Source: CAD feature listing. Evaluate the final solid. Frame: model axes, mm. Coordinates: 2 decimals unless noted, no trailing zeros. Order: outer loops, then holes, each group sorted by start corner. A loop starts at its lowest first (then second) coordinate and runs counter-clockwise, first axis right, second up. Notation, with made-up numbers: (21, -37.75) -> (44, -37.75) arc R20 ccw to (44, -27.75) -> close; hole circle Ø7 at (-6, 30). An arc over 180 degrees is marked (long way). Write item = value, one per line. Start each with the question number.
Item 1: Ray query, line 1 along X through (y, z) = (17.5, 0.65); line 2 along X through (y, z) = (18, 2.1). Return the intervals inside material, ascending. Write a range as [from, to].
Item 2: Contact query for flat-ended pins moving along their axis: pin 1 (6 mm diameter, centred on x = -17, y = 13, fed in from -Z); pin 2 (0.8 mm diameter, centred on y = 0, z = 2, fed in from +X); pin 3 (1.4 mm diameter, centred on x = 21, z = 1, fed in from -Y); pin 4 (1.4 mm diameter, centred on x = -22, z = 1.5, fed in from -Y). Output: stop coordinate, or through.
Item 3: Section query B-B (y = 21). Output: boundary loops of the cut face in (x, z), then the cut area to 3 significant figures.
Item 4: Section query A-A (z = 0.6). Output: boundary loops of the cut face in (x, y).
Item 5: Section query D-D (y = -0.5). Output: boundary loops of the cut face in (x, z), then the cut area to 3 significant figures.
Item 6: Section query C-C (x = -17). Output: boundary loops of the cut face in (y, z), then the cut area to 3 significant figures.
```python
from build123d import *

# Parameters (mm, degrees)
CROQUIS1_R              = 25
SALIENTE_EXTRUIR1_DEPTH = 2.8
CROQUIS2_W              = 2.8
CROQUIS2_H              = 18
CORTAR_EXTRUIR1_DEPTH   = 3.8
MATRIZC1_COUNT          = 4


with BuildPart() as part:
    # Croquis1 → Saliente-Extruir1 (new body)
    with BuildSketch(Plane.XY):
        Circle(CROQUIS1_R)
    extrude(amount=SALIENTE_EXTRUIR1_DEPTH)

    # Croquis2 → Cortar-Extruir1 (cut, through all)
    with BuildSketch(Plane.XY):
        with Locations((0, 25)):
            Rectangle(CROQUIS2_W, CROQUIS2_H)
    cortar_extruir1 = extrude(amount=CORTAR_EXTRUIR1_DEPTH, mode=Mode.SUBTRACT)

    # MatrizC1: Cortar-Extruir1 ×4 about axis
    matrizc1_axis = Axis((0, 0, 0), (0, 0, 1))
    for i in range(1, MATRIZC1_COUNT):
        add(cortar_extruir1.rotate(matrizc1_axis, i * 360 / MATRIZC1_COUNT), mode=Mode.SUBTRACT)


solid = part.part
```
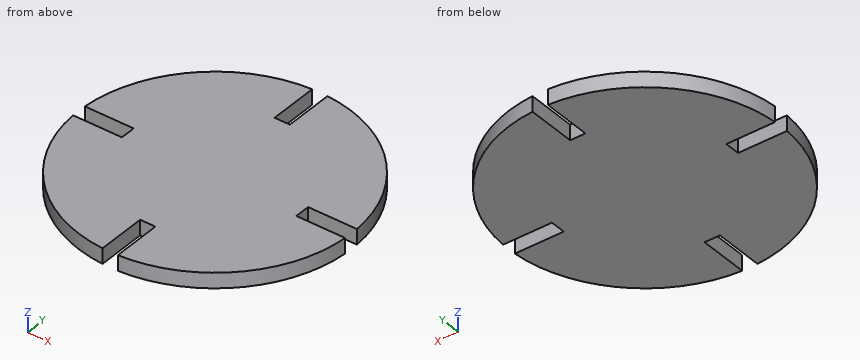
Computed:
q1.line_1 = [-17.85, -1.4], [1.4, 17.85]
q1.line_2 = [-17.35, -1.4], [1.4, 17.35]
q2.pin_1 = 0
q2.pin_2 = 16
q2.pin_3 = -14.59
q2.pin_4 = -13.09
q3.outline = (-13.56, 0) -> (-1.4, 0) -> (-1.4, 2.8) -> (-13.56, 2.8) -> close; (1.4, 0) -> (13.56, 0) -> (13.56, 2.8) -> (1.4, 2.8) -> close
q3.area = 68.1 mm^2
q4.outline = (-24.96, -1.4) arc R25 ccw to (-1.4, -24.96) -> (-1.4, -16) -> (1.4, -16) -> (1.4, -24.96) arc R25 ccw to (24.96, -1.4) -> (16, -1.4) -> (16, 1.4) -> (24.96, 1.4) arc R25 ccw to (1.4, 24.96) -> (1.4, 16) -> (-1.4, 16) -> (-1.4, 24.96) arc R25 ccw to (-24.96, 1.4) -> (-16, 1.4) -> (-16, -1.4) -> close
q5.outline = (-16, 0) -> (16, 0) -> (16, 2.8) -> (-16, 2.8) -> close
q5.area = 89.6 mm^2
q6.outline = (-18.33, 0) -> (-1.4, 0) -> (-1.4, 2.8) -> (-18.33, 2.8) -> close; (1.4, 0) -> (18.33, 0) -> (18.33, 2.8) -> (1.4, 2.8) -> close
q6.area = 94.8 mm^2
